Model file for the job. Use its own axes, mm. Round coordinates to 2 decimals unless told otherwise and drop trailing zeros. Order: outer loops, then holes, each group sorted by start corner. A loop starts at its lowest first (then second) coordinate and runs counter-clockwise, first axis right, second up. Notation, with made-up numbers: (-5.5, 43) - (53.5, 43) arc R20 ccw to (53.5, 82) - close; hole circle Ø6 at (6, 26). An arc over 180 degrees is marked (long way). Put each result on its own line as item: value. Start each with the question number.
Item 1: Mould opens along Y. For faces 1 (the face through (-0.38, 75.54, 3.04)), 2 (the face through (0, 36, 6)) say: pulls with the +Y half, pulls with the -Y half, needs draft (parallel to the pull), parting line crosses it, or undercut.
Item 2: Saw through at A-A on y = 0. List the corners of the cut face in (x, z), plus the area to 3 significant figures.
Item 3: Pin check, flat tip, straight feed: pin 1 Ø3 at (y, z) = (72, 2.5) entering from +X. Stop position of the tip, or through.
Item 4: Saw through at B-B on z = 2.6. State how many separate pieces and enclosed holes the cut face has, plus the area to 3 significant figures.
Item 5: Probe probe 1 along Y at (x, z) = (7.25, 2.05); probe 2 along Y at (x, z) = (2.75, 1.65); probe 3 along X at (y, z) = (19, 3.5). List the from-to ranges inside material, lowest first.
Item 6: Saw through at D-D on y = 77.25. List the corners of the cut face in (x, z).
Item 7: Saw through at C-C on x = -3. List the corners of the cut face in (y, z), plus the area to 3 significant figures.
```python
from build123d import *

# Parameters (mm, degrees)
SKETCH1_R           = 12.5
SKETCH1_R_2         = 1.5
BOSS_EXTRUDE1_DEPTH = 6
SKETCH2_R           = 4
SKETCH2_R_2         = 1.75
CUT_EXTRUDE1_DEPTH  = 84.657037959


with BuildPart() as part:
    # Sketch1 → Boss-Extrude1 (new body)
    with BuildSketch(Plane.XY):
        with BuildLine():
            ThreePointArc((-12.468548805, 0.886166287), (-2.14802756, 12.314056099), (11.432131685, 5.05533037))
            ThreePointArc((11.432131685, 5.05533037), (8.045519539, 19.668908158), (10.280253267, 34.502375816))
            ThreePointArc((10.280253267, 34.502375816), (7.365201971, 34.999999986), (10.280253258, 35.497624211))
            ThreePointArc((10.280253258, 35.497624211), (8.045519539, 50.331091856), (11.432131685, 64.944669631))
            ThreePointArc((11.432131685, 64.944669631), (-2.148028371, 57.685944043), (-12.468548922, 69.113835355))
            ThreePointArc((-12.468548922, 69.113835355), (-11.560587189, 52.067656989), (-11.257806268, 35))
            ThreePointArc((-11.257806268, 35), (-11.56058716, 17.932343833), (-12.468548805, 0.886166287))
        make_face()
        with Locations((0, 70)):
            Circle(SKETCH1_R)
        with Locations((8.865201971, 35)):
            Circle(SKETCH1_R_2)
        Circle(SKETCH1_R)
    extrude(amount=BOSS_EXTRUDE1_DEPTH)

    # Sketch2 → Cut-Extrude1 (cut, through all)
    with BuildSketch(Plane.XY.offset(6)):
        with Locations((0, 70)):
            Circle(SKETCH2_R)
        Circle(SKETCH2_R)
        with Locations((0, 7.25)):
            Circle(SKETCH2_R_2)
        with Locations((7.25, 0)):
            Circle(SKETCH2_R_2)
        with Locations((0, -7.25)):
            Circle(SKETCH2_R_2)
        with Locations((-7.25, 0)):
            Circle(SKETCH2_R_2)
        with Locations((0, 77.25)):
            Circle(SKETCH2_R_2)
        with Locations((7.25, 70)):
            Circle(SKETCH2_R_2)
        with Locations((0, 62.75)):
            Circle(SKETCH2_R_2)
        with Locations((-7.25, 70)):
            Circle(SKETCH2_R_2)
    extrude(amount=-CUT_EXTRUDE1_DEPTH, mode=Mode.SUBTRACT)


solid = part.part
```
Results found:
1. face 1: undercut
1. face 2: needs draft
2. outline: (-12.5, 0) - (-9, 0) - (-9, 6) - (-12.5, 6) - close; (-5.5, 0) - (-4, 0) - (-4, 6) - (-5.5, 6) - close; (4, 0) - (5.5, 0) - (5.5, 6) - (4, 6) - close; (9, 0) - (12.5, 0) - (12.5, 6) - (9, 6) - close
2. area: 60.0 mm²
3. pin 1: stops at x = 12.49
4. separate pieces: 1
4. enclosed holes: 10
4. area: 1,790 mm²
5. probe 1: y = -10.18 to -1.75, 1.75 to 68.25, 71.75 to 80.18
5. probe 2: y = -12.19 to -2.9, 2.9 to 67.1, 72.9 to 82.19
5. probe 3: x = -11.52 to 8.08
6. outline: (-10.18, 0) - (-1.75, 0) - (-1.75, 6) - (-10.18, 6) - close; (1.75, 0) - (10.18, 0) - (10.18, 6) - (1.75, 6) - close
7. outline: (-12.13, 0) - (-2.65, 0) - (-2.65, 6) - (-12.13, 6) - close; (2.65, 0) - (67.35, 0) - (67.35, 6) - (2.65, 6) - close; (72.65, 0) - (82.13, 0) - (82.13, 6) - (72.65, 6) - close
7. area: 502 mm²
